Autodesk Inventor part; units mm, degrees
ref_plane "РабПлоскость1" through (0, 0, -68.5) normal (0, 0, 1) x (1, 0, 0)
ref_plane "YZ Plane" through (0, 0, 0) normal (1, 0, 0) x (0, 1, 0)
ref_plane "XZ Plane" through (0, 0, 0) normal (0, 1, 0) x (-1, 0, 0)
sketch "Эскиз1" plane through (0, 0, 0) normal (0, 1, 0) x (-1, 0, 0)
  line L0 (0, 0) -> (148, 0)
  line L1 (148, 0) -> (148, -137)
  line L2 (148, -137) -> (0, -137)
  line L3 (0, -137) -> (0, 0)
  line L4 (10, -10) -> (138, -10)
  line L5 (138, -10) -> (138, -127)
  line L6 (138, -127) -> (10, -127)
  line L7 (10, -127) -> (10, -10)
  line L8 (0, 0) -> (5.5771, 0)
  dimension "d0" = 148
  dimension "d2" = 10
  dimension "d3" = 10
  dimension "d4" = 10
  dimension "d5" = 10
  dimension "d8" = 117
extrude "Выдавливание1" add sketch "Эскиз1" along normal blind 25
sketch "Эскиз2" plane through (0, 25, 0) normal (0, 1, 0) x (1, 0, 0)
  line L0 (0, 0) -> (0, 137)
  line L1 (-148, 0) -> (0, 0)
  line L2 (0, 5) -> (-148, 5)
  line L3 (-148, 137) -> (-148, 0)
  line L4 (-143, 0) -> (-148, 0)
  line L5 (-143, 0) -> (-143, 137)
  line L6 (0, 137) -> (-148, 137)
  circle A0 centre (-143, 5) radius 2.5
  dimension "d9" = 5
  dimension "d12" = 5
  dimension "d20" = 5
extrude "Выдавливание2" cut sketch "Эскиз2" against normal through all contours A0 L5 L2 | L2 L5 A0 | A0 L2 L5 | L2 A0 L5
sketch "Эскиз6" plane through (0, 25, 0) normal (0, 1, 0) x (1, 0, 0)
  line L0 (-98, 137) -> (-98, 127)
  line L1 (-138, 127) -> (-10, 127)
  line L2 (-148, 137) -> (-148, 0)
  line L3 (-98, 127) -> (-101, 127)
  line L4 (-101, 137) -> (-101, 127)
  line L5 (-101, 137) -> (-98, 137)
  line L6 (0, 137) -> (-148, 137)
  point P0 (0, 0)
  dimension "d46" = 50
  dimension "d47" = 6
  dimension "d86" = 10
revolve "Вращение3" cut sketch "Эскиз6" angle 360 about axis through (-98, 25, -137) along (0, 0, 1)
sketch "Эскиз8" plane through (0, 25, 0) normal (0, 1, 0) x (1, 0, 0)
  circle A0 centre (-143, 5) radius 2.5
  line L0 (-143, 5) -> (-48, 5)
  circle A1 centre (-5, 5) radius 2.5
  line L1 (0, 0) -> (0, 137)
  dimension "d56" = 5
  dimension "d57" = 5
extrude "Выдавливание4" cut sketch "Эскиз8" against normal through all contours A1
sketch "Эскиз9" plane through (0, 25, 0) normal (0, 1, 0) x (1, 0, 0)
  circle A0 centre (-5, 5) radius 2.5
  line L0 (-5, 5) -> (-5, 137)
  line L1 (0, 137) -> (-148, 137)
  circle A1 centre (-5, 132) radius 2.5
  point P0 (0, 0)
  point P1 (0, 137)
  point P2 (-85.5, 143)
  dimension "d60" = 5
  dimension "d61" = 5
extrude "Выдавливание5" cut sketch "Эскиз9" against normal through all contours A1 L0 | L0 A1
sketch "Эскиз10" plane through (0, 25, 0) normal (0, 1, 0) x (1, 0, 0)
  circle A0 centre (-143, 5) radius 2.5
  line L0 (-143, 5) -> (-143, 137)
  line L1 (-148, 137) -> (0, 137)
  circle A1 centre (-5, 132) radius 2.5
  line L2 (-5, 132) -> (-148, 132)
  line L3 (-148, 0) -> (-148, 137)
  circle A2 centre (-143, 132) radius 2.5
  point P0 (0, 0)
  dimension "d64" = 5
extrude "Выдавливание6" cut sketch "Эскиз10" against normal through all contours A2 L2 L0 | L0 L2 A2 | L2 A2 L0 | L0 A2 L2
sketch "Эскиз11" plane through (-10, 0, -10) normal (0, 0, -1) x (-1, 0, 0)
  line L0 (0, 25) -> (128, 25)
  circle A0 centre (88, 25) radius 18.5
  line L1 (128, 0) -> (0, 0)
  circle A1 centre (88, 6.5) radius 2.4
  line L2 (88, 25) -> (88, 6.5)
  line L3 (88, 25) -> (69.5, 25)
  point P0 (-10, 0)
  point P1 (-10, 25)
  point P2 (138, 25)
  dimension "d67" = 37
  dimension "d69" = 4.8
  dimension "d79" = 50
  dimension "d85" = 90
extrude "Выдавливание7" cut sketch "Эскиз11" against normal through all contours A1 L2 A0 | A0 A1 | A1 A0 L2
pattern_linear "Прямоуг.массив3" count 2 spacing -73 along (-1, 0, 0) of "Выдавливание7"
ref_plane "РабПлоскость1" through (0, 0, -68.5) normal (0, 0, 1) x (1, 0, 0)
mirror "Зеркальное отражение1" about plane through (0, 0, -68.5) normal (0, 0, 1) of "Прямоуг.массив3"
sketch "Эскиз14" plane through (0, 0, -137) normal (0, 0, -1) x (-1, 0, 0)
  arc A0 (95, 25) -> (101, 25) centre (98, 25) ccw
  line L0 (113, 9) -> (113, 25)
  line L1 (138, 25) -> (101, 25)
  line L2 (113, 25) -> (28, 25)
  line L3 (0, 25) -> (95, 25)
  line L4 (28, 25) -> (28, 9)
  line L5 (28, 9) -> (113, 9)
  point P0 (0, 0)
  point P1 (148, 25)
  dimension "d89" = 85
  dimension "d90" = 16
  dimension "d91" = 35
extrude "Выдавливание8" cut sketch "Эскиз14" against normal blind 3 contours A0 L1 L0 L5 L4 L2
sketch "Эскиз15" plane through (0, 0, -134) normal (0, 0, -1) x (-1, 0, 0)
  arc A0 (95, 25) -> (101, 25) centre (98, 25) ccw
  line L0 (148, 25) -> (0, 25)
  line L1 (113, 9) -> (107, 9)
  line L2 (113, 9) -> (28, 9)
  line L3 (107, 9) -> (107, 16)
  circle A1 centre (107, 16) radius 1.5
  point P0 (0, 0)
  dimension "d98" = 6
  dimension "d99" = 7
  dimension "d100" = 3
extrude "Выдавливание9" cut sketch "Эскиз15" against normal up to next contours A1
sketch "Эскиз16" plane through (0, 0, -134) normal (0, 0, -1) x (-1, 0, 0)
  line L0 (113, 9) -> (28, 9)
  circle A0 centre (107, 16) radius 1.5
  line L1 (107, 16) -> (74, 16)
  circle A1 centre (74, 16) radius 1.5
  point P0 (0, 0)
  dimension "d106" = 33
  dimension "d107" = 3
extrude "Выдавливание10" cut sketch "Эскиз16" against normal up to next contours A1
sketch "Эскиз17" plane through (0, 0, -134) normal (0, 0, -1) x (-1, 0, 0)
  circle A0 centre (74, 16) radius 1.5
  circle A1 centre (74, 16) radius 3.7
  point P0 (0, 0)
  dimension "d110" = 7.4
extrude "Выдавливание11" cut sketch "Эскиз17" against normal blind 2
sketch "Эскиз18" plane through (0, 0, -134) normal (0, 0, -1) x (-1, 0, 0)
  circle A0 centre (107, 16) radius 1.5
  circle A1 centre (107, 16) radius 3.7
  point P0 (0, 0)
  dimension "d113" = 7.4
extrude "Выдавливание12" cut sketch "Эскиз18" against normal blind 2
sketch "Эскиз19" plane through (0, 0, -134) normal (0, 0, -1) x (-1, 0, 0)
  arc A0 (82, 20) -> (88, 20) centre (85, 20) ccw
  line L0 (113, 9) -> (28, 9)
  line L1 (113, 25) -> (113, 9)
  line L2 (10, 25) -> (138, 25)
  line L3 (82, 20) -> (82, 25)
  line L4 (88, 20) -> (88, 25)
  point P0 (0, 0)
  dimension "d121" = 6
  dimension "d123" = 25
  dimension "d124" = 11
extrude "Выдавливание13" cut sketch "Эскиз19" against normal blind 2
properties part number "Корпус низ"
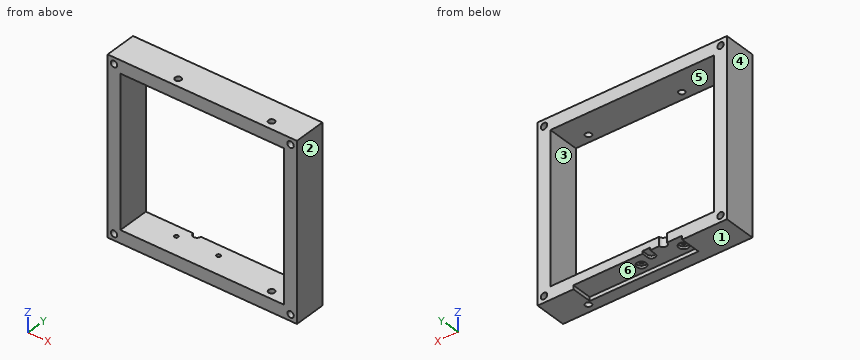
Geometry check sheet. Reference: the model listing, model coordinates, mm. Face numbers are marked on the shaded views. A direction names the side the tool comes from. Give positions to 0.01 mm unless a question says otherwise; leave off trailing zeros. Loops run counter-clockwise (first coordinate to the right, second up) from the corner with the lowest first, then second, coordinate; pieces in that order, holes last. Notation, with made-up numbers: M -14.5,55.25 L 1.5,55.25 A12 cw 1.5,69.25 Z; hole C 20,-5.75 d8. An arc over 180 degrees is marked long. Answer as a JSON object with one key per item and string values. Group by question number.
Item 1: Sectioned sample at B-B on x = -85. Record the boundary of the cut face in (y, z), plus the area to 3 significant figures.
Item 2: Sectioned sample at A-A on z = -48.5. Record the boundary of the cut face in (x, y).
Item 3: Material ranges on L1, parallel to Z at x = -5, y = 19; L2, parallel to Z at x = -131, y = 23.75, recorded low to high.
Item 4: Sectioned sample at D-D on x = -5. Record the boundary of the cut face in (y, z), plus the area to 4 significant figures.
Item 5: Access from +Z, -Z, +X, -X, +Y, -Y to the whole of each face (thin tool, end or side, straight path). Record for the marked faces 4, 5 and 6.
Item 6: Sectioned sample at C-C on y = 6.5. Record the boundary of the cut face in (x, z), plus the area to 3 significant figures.
Item 7: Mould release check, pull along Z, two halves, no side actions. Record for the marked faces 1, 2 and 3: pulls with the +Z half, pulls with the -Z half, needs draft (parallel to the pull), parting line crosses it, or undercut.
Item 8: Gauge pin test, flat ends, axial feed: pin 1 (0.9 mm diameter, centred on x = -90, z = -136, fed in from +Y); pin 2 (6 mm diameter, centred on x = -72.5, y = 17.5, fed in from -Z). Record the tip position at first contact, or that the pin passes through.
Findings below:
{
 "1": {"outline": "M 0,-137 L 9,-137 L 9,-134 L 17,-134 L 17,-132 L 25,-132 L 25,-127 L 0,-127 Z; M 0,-10 L 25,-10 L 25,0 L 0,0 Z", "area": "436 mm2"},
 "2": {"outline": "M -148,0 L -138,0 L -138,25 L -148,25 Z; M -10,0 L 0,0 L 0,25 L -10,25 Z"},
 "3": {"L1": "-137 to -134.5, -129.5 to -7.5, -2.5 to 0", "L2": "-137 to -127, -10 to 0"},
 "4": {"outline": "M 0,-137 L 25,-137 L 25,-134.5 L 0,-134.5 Z; M 0,-129.5 L 25,-129.5 L 25,-7.5 L 0,-7.5 Z; M 0,-2.5 L 25,-2.5 L 25,0 L 0,0 Z", "area": "3,175 mm2"},
 "5": {"face 4": "+Z, -Z, -X, +Y, -Y", "face 5": "+Y, -Y", "face 6": "-Z, +Y"},
 "6": {"outline": "M -148,-137 L -27.4,-137 L -27.4,-127 L -138,-127 L -138,-10 L -100.4,-10 L -100.4,0 L -148,0 Z; M -95.6,-10 L -27.4,-10 L -27.4,0 L -95.6,0 Z; M -22.6,-137 L 0,-137 L 0,0 L -22.6,0 L -22.6,-10 L -10,-10 L -10,-127 L -22.6,-127 Z; hole C -143,-132 d5; hole C -143,-5 d5; hole C -5,-132 d5; hole C -5,-5 d5", "area": "5,080 mm2"},
 "7": {"face 1": "pulls with the -Z half", "face 2": "needs draft", "face 3": "undercut"},
 "8": {"pin 1": "y = 9", "pin 2": "z = -134"}
}
